Input: part model. Units: mm. Frame: model coordinates. A direction names the side the tool comes from. Coordinates: 2 decimals unless noted, no trailing zeros. Use a Markdown table: item, result. Add a question column.
Q1. Set-up query: faces 5 (the face through (94, 4, 72.7)), 6 (the face through (4, 7, 64.1)), 7 (the face through (94, 4, 52.7)), 8 (the face through (8, 9, 97.5)). Return all of +Z, -Z, +X, -X, +Y, -Y with unobstructed straight access to the full face (end or side cutting, diameter ignored); none if empty.
Q2. Mould query, pull axis X, two halves, no side actions, for faces 1 (the face through (56.654, -3.944, 39.761)), 2 (the face through (3, 6, 64.9)), 3 (the face through (0, 5, 50)), 4 (the face through (84.4, -2, 76)). Classes: released by +X, released by -X, zero draft, split by the parting line, or undercut.
Q3. Material intervals for probe 1 along X at (y, z) = (5.75, 21); probe 2 along Z at (x, y) = (94.8, 0.95); probe 3 along X at (y, z) = (11, 13), sorted ascending. Write a range as from..to.
Q4. Pin query (flat end, axial travel): P1, Ø5, axis at y = 3.5, z = 36.5, coming from the +X side; P2, Ø2, axis at x = 41, z = 53, coming from the -Y side; P3, Ø10, axis at y = 8, z = 63.5, coming from the -X side; P4, Ø5, axis at x = 74.5, y = 4.5, coming from the +Z side. Return the tip coordinate at first contact, or that it passes through.
from build123d import *

# Parameters (mm, degrees)
SKETCH_1_W       = 99
SKETCH_1_H       = 99
SKETCH_1_R       = 1.05
EXTRUDE_1_DEPTH  = 1.6
SKETCH_2_W       = 7.6
SKETCH_2_H       = 23.2
SKETCH_2_W_2     = 13.1
SKETCH_2_H_2     = 17.5
SKETCH_2_W_3     = 21.3
SKETCH_2_H_3     = 16
EXTRUDE_2_DEPTH  = 14
SKETCH_3_W       = 8.6
SKETCH_3_H       = 6.9
EXTRUDE_3_DEPTH  = 3
SKETCH_4_W       = 20.1
SKETCH_4_H       = 6
SKETCH_4_W_2     = 13.8
SKETCH_4_H_2     = 14.3
EXTRUDE_4_DEPTH  = 2
SKETCH_5_W       = 11.9
SKETCH_5_H       = 10.1
SKETCH_5_W_2     = 6
SKETCH_5_H_2     = 13
EXTRUDE_5_DEPTH  = 7
SKETCH_6_W       = 9
SKETCH_6_H       = 39.2
EXTRUDE_6_DEPTH  = 11
SKETCH_7_W       = 6.5
SKETCH_7_H       = 16
EXTRUDE_7_DEPTH  = 8
SKETCH_8_W       = 9
SKETCH_8_H       = 16
SKETCH_8_H_2     = 8.4
SKETCH_8_W_2     = 4.5
SKETCH_8_H_3     = 3.7
EXTRUDE_8_DEPTH  = 4
SKETCH_9_W       = 5.2
SKETCH_9_H       = 12
EXTRUDE_9_DEPTH  = 6
SKETCH_10_R      = 7.5
SKETCH_10_W      = 14.6
SKETCH_10_H      = 6
EXTRUDE_10_DEPTH = 4
SKETCH_11_W      = 4
SKETCH_11_H      = 11.6
SKETCH_11_W_2    = 16.2
SKETCH_11_H_2    = 6
EXTRUDE_11_DEPTH = 2
SKETCH_12_W      = 7.5
SKETCH_12_H      = 8.9
SKETCH_12_W_2    = 3.5
SKETCH_12_H_2    = 9.1
EXTRUDE_12_DEPTH = 3
SKETCH_13_W      = 7.4
SKETCH_13_H      = 21.9
SKETCH_13_W_2    = 6.9
EXTRUDE_13_DEPTH = 6.4
SKETCH_14_R      = 7.5
EXTRUDE_14_DEPTH = 8


with BuildPart() as part:
    # 草图1 → 凸台-拉伸1 (new body)
    with BuildSketch(Plane(origin=(0, 0, 0), x_dir=(1, 0, 0), z_dir=(0, 1, 0))):
        with Locations((49.5, -49.5)):
            Rectangle(SKETCH_1_W, SKETCH_1_H)
        with Locations(Location((21.8, -26.8, 0), (0, 0, 270))):
            Circle(SKETCH_1_R, mode=Mode.SUBTRACT)
        with Locations(Location((94.8, -26.8, 0), (0, 0, 270))):
            Circle(SKETCH_1_R, mode=Mode.SUBTRACT)
        with Locations(Location((21.8, -94.8, 0), (0, 0, 270))):
            Circle(SKETCH_1_R, mode=Mode.SUBTRACT)
        with Locations(Location((94.8, -94.8, 0), (0, 0, 270))):
            Circle(SKETCH_1_R, mode=Mode.SUBTRACT)
        with Locations(Location((8.7, -65.7, 0), (0, 0, 270))):
            Circle(SKETCH_1_R, mode=Mode.SUBTRACT)
        with Locations(Location((81.9, -4.6, 0), (0, 0, 270))):
            Circle(SKETCH_1_R, mode=Mode.SUBTRACT)
        with Locations(Location((96.3, -55.2, 0), (0, 0, 270))):
            Circle(SKETCH_1_R, mode=Mode.SUBTRACT)
        with Locations(Location((20, -12, 0), (0, 0, 270))):
            Circle(SKETCH_1_R, mode=Mode.SUBTRACT)
        with Locations(Location((71.4, -77.5, 0), (0, 0, 270))):
            Circle(SKETCH_1_R, mode=Mode.SUBTRACT)
    extrude(amount=EXTRUDE_1_DEPTH)

    # 草图2 → 凸台-拉伸2 (add)
    with BuildSketch(Plane(origin=(0, 1.6, 0), x_dir=(1, 0, 0), z_dir=(0, 1, 0))):
        with Locations((92.9, -9.6)):
            Rectangle(SKETCH_2_W, SKETCH_2_H)
        with Locations((75.6, -9.6)):
            Rectangle(SKETCH_2_W, SKETCH_2_H)
        with Locations((55.15, -6.75)):
            Rectangle(SKETCH_2_W_2, SKETCH_2_H_2)
        with Locations((8.55, -89.5)):
            Rectangle(SKETCH_2_W_3, SKETCH_2_H_3)
    extrude(amount=EXTRUDE_2_DEPTH)

    # 草图3 → 凸台-拉伸3 (add)
    with BuildSketch(Plane(origin=(0, 1.6, 0), x_dir=(1, 0, 0), z_dir=(0, 1, 0))):
        with Locations((40.4, -3.45)):
            Rectangle(SKETCH_3_W, SKETCH_3_H)
    extrude(amount=EXTRUDE_3_DEPTH)

    # 草图4 → 凸台-拉伸4 (add)
    with BuildSketch(Plane(origin=(0, 1.6, 0), x_dir=(1, 0, 0), z_dir=(0, 1, 0))):
        with Locations((24.45, -3)):
            Rectangle(SKETCH_4_W, SKETCH_4_H)
        with Locations((89.2, -35.55)):
            Rectangle(SKETCH_4_W_2, SKETCH_4_H_2)
    extrude(amount=EXTRUDE_4_DEPTH)

    # 草图5 → 凸台-拉伸5 (add)
    with BuildSketch(Plane(origin=(0, 1.6, 0), x_dir=(1, 0, 0), z_dir=(0, 1, 0))):
        with Locations((5.95, -18.95)):
            Rectangle(SKETCH_5_W, SKETCH_5_H)
        with Locations((10.2, -73.7)):
            Rectangle(SKETCH_5_W_2, SKETCH_5_H_2)
    extrude(amount=EXTRUDE_5_DEPTH)

    # 草图6 → 凸台-拉伸6 (add)
    with BuildSketch(Plane(origin=(0, 1.6, 0), x_dir=(1, 0, 0), z_dir=(0, 1, 0))):
        with Locations((4.5, -44.5)):
            Rectangle(SKETCH_6_W, SKETCH_6_H)
    extrude(amount=EXTRUDE_6_DEPTH)

    # 草图7 → 凸台-拉伸7 (add)
    with BuildSketch(Plane(origin=(0, 1.6, 0), x_dir=(1, 0, 0), z_dir=(0, 1, 0))):
        with Locations((3.25, -72.9)):
            Rectangle(SKETCH_7_W, SKETCH_7_H)
    extrude(amount=EXTRUDE_7_DEPTH)

    # 草图8 → 凸台-拉伸8 (add)
    with BuildSketch(Plane(origin=(0, 1.6, 0), x_dir=(1, 0, 0), z_dir=(0, 1, 0))):
        with Locations((94.5, -64.7)):
            Rectangle(SKETCH_8_W, SKETCH_8_H)
        with Locations((94.5, -48.5)):
            Rectangle(SKETCH_8_W, SKETCH_8_H_2)
        with Locations((20.75, -22.25)):
            Rectangle(SKETCH_8_W_2, SKETCH_8_H_3)
    extrude(amount=EXTRUDE_8_DEPTH)

    # 草图9 → 凸台-拉伸9 (add)
    with BuildSketch(Plane.XZ):
        with Locations((95.8, 87.4)):
            Rectangle(SKETCH_9_W, SKETCH_9_H)
    extrude(amount=EXTRUDE_9_DEPTH)

    # 草图10 → 凸台-拉伸10 (add)
    with BuildSketch(Plane.XZ):
        with Locations(Location((85.4, 55.4, 0), (0, 0, 90))):
            Circle(SKETCH_10_R)
        with Locations((91.7, 76.5)):
            Rectangle(SKETCH_10_W, SKETCH_10_H)
    extrude(amount=EXTRUDE_10_DEPTH)

    # 草图11 → 凸台-拉伸11 (add)
    with BuildSketch(Plane.XZ):
        with Locations((95.7, 46)):
            Rectangle(SKETCH_11_W, SKETCH_11_H)
        with Locations((26.3, 3)):
            Rectangle(SKETCH_11_W_2, SKETCH_11_H_2)
    extrude(amount=EXTRUDE_11_DEPTH)

    # 草图12 → 凸台-拉伸12 (add)
    with BuildSketch(Plane.XZ):
        with Locations((95.25, 34.05)):
            Rectangle(SKETCH_12_W, SKETCH_12_H)
        with Locations((37.85, 38.85)):
            Rectangle(SKETCH_12_W_2, SKETCH_12_H_2)
    extrude(amount=EXTRUDE_12_DEPTH)

    # 草图13 → 凸台-拉伸13 (add)
    with BuildSketch(Plane.XZ):
        with Locations((41.7, 77.45)):
            Rectangle(SKETCH_13_W, SKETCH_13_H)
        with Locations((16.25, 55.25)):
            Rectangle(SKETCH_13_W_2, SKETCH_13_H)
    extrude(amount=EXTRUDE_13_DEPTH)

    # 草图14 → 凸台-拉伸14 (add)
    with BuildSketch(Plane.XZ):
        with Locations(Location((50, 36.3, 0), (0, 0, 90))):
            Circle(SKETCH_14_R)
    extrude(amount=EXTRUDE_14_DEPTH)


solid = part.part
Values follow:
| question | item | result |
|---|---|---|
| 1 | face 5 | +Z, +X, +Y |
| 1 | face 6 | -X, +Y |
| 1 | face 7 | +X, +Y |
| 1 | face 8 | +Z, +X, -X, +Y |
| 2 | face 1 | undercut |
| 2 | face 2 | zero draft |
| 2 | face 3 | released by -X |
| 2 | face 4 | undercut |
| 3 | probe 1 | 0..11.9, 71.8..79.4, 89.1..96.7 |
| 3 | probe 2 | 0..25.75, 27.85..93.75, 95.85..99 |
| 3 | probe 3 | 48.6..61.7, 71.8..79.4, 89.1..96.7 |
| 4 | P1 | x = 99 |
| 4 | P2 | y = 0 |
| 4 | P3 | x = 0 |
| 4 | P4 | z = 21.2 |
